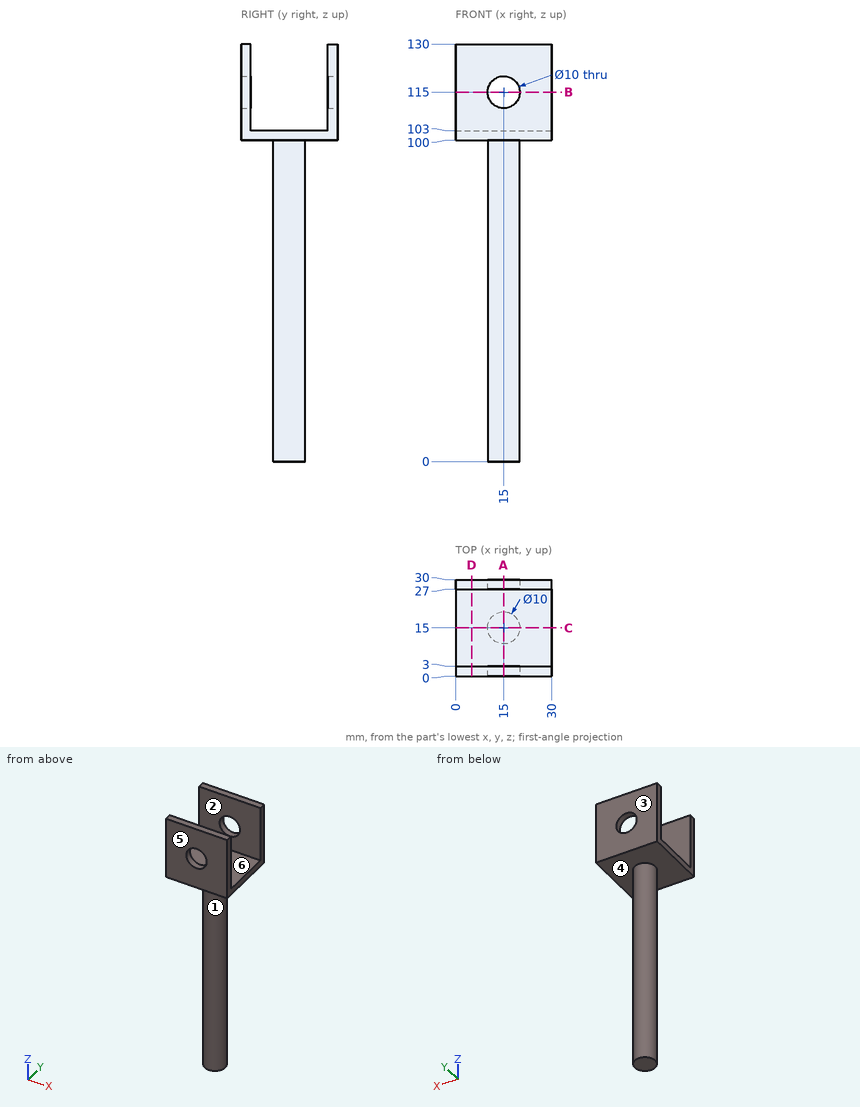
Part print with two shaded views. Sizes in mm from the minimum x, y, z corner. A direction names the side the tool comes from. Round coordinates to 2 decimals unless told otherwise and drop trailing zeros. Loops run counter-clockwise (first coordinate to the right, second up) from the corner with the lowest first, then second, coordinate; pieces in that order, holes last.
1. Slice it at C-C (y = 15). Give the cut face in (x, z), and give its area (3 significant figures).
Solutions:
outline: (0, 100) - (10, 100) - (10, 0) - (20, 0) - (20, 100) - (30, 100) - (30, 103) - (0, 103) - close
area: 1,090 mm2
2. Slice it at B-B (z = 115). Give the cut face in (x, y).
Solutions:
outline: (0, 0) - (10, 0) - (10, 3) - (0, 3) - close; (0, 27) - (10, 27) - (10, 30) - (0, 30) - close; (20, 0) - (30, 0) - (30, 3) - (20, 3) - close; (20, 27) - (30, 27) - (30, 30) - (20, 30) - close
3. Slice it at A-A (x = 15). Give the cut face in (y, z), and give its area (3 significant figures).
Solutions:
outline: (0, 100) - (10, 100) - (10, 0) - (20, 0) - (20, 100) - (30, 100) - (30, 110) - (27, 110) - (27, 103) - (3, 103) - (3, 110) - (0, 110) - close; (0, 120) - (3, 120) - (3, 130) - (0, 130) - close; (27, 120) - (30, 120) - (30, 130) - (27, 130) - close
area: 1,190 mm2
4. Two-plate mould, pull along Y, no slides. Class the marked faces 4, 5 and 6: pulls with the +Y half, pulls with the -Y half, needs draft (parallel to the pull), parting line crosses it, or undercut.
Solutions:
face 4: needs draft
face 5: pulls with the -Y half
face 6: undercut
5. Slice it at D-D (x = 5). Give the cut face in (y, z).
Solutions:
outline: (0, 100) - (30, 100) - (30, 130) - (27, 130) - (27, 103) - (3, 103) - (3, 130) - (0, 130) - close
6. Flat gauge pins, fed straight in: pin 1 (7 mm diameter, centred on x = 14, y = 17, fed in from +Z); pin 2 (10 mm diameter, centred on y = 21, z = 24, fed in from -X); pin 3 (8 mm diameter, centred on x = 16.5, z = 57.5, fed in from +Y). Where does each tip first touch, or does it go through?
Solutions:
pin 1: stops at z = 103
pin 2: stops at x = 10.1
pin 3: stops at y = 20
7. Drill centre lines: line 1 along X through (y, z) = (28.7, 115); line 2 along Z through (x, y) = (15, 1.75); line 3 along Z through (x, y) = (1.5, 10.75). Where is each one in solid material? Low to high.
Solutions:
line 1: x = 0 to 10, 20 to 30
line 2: z = 100 to 110, 120 to 130
line 3: z = 100 to 103
8. 3-axis set-ups, long thin cutter, end or side, ignore diameter. For the marked faces 1, 2 and 3: which of +Z, -Z, +X, -X, +Y, -Y reach the whole face in a straight line?
Solutions:
face 1: -Z
face 2: +Z, +X, -X
face 3: +Z, -Z, +X, -X, +Y
